from build123d import *

# Parameters (mm, degrees)
SKETCH_1_W                = 44.5
SKETCH_1_H                = 40
EXTRUDE_1_DEPTH           = 9
SKETCH_2_W                = 40.5
SKETCH_2_H                = 7.5
CUT_EXTRUDE_1_DEPTH       = 47.64828507
CUT_EXTRUDE_2_REACH       = 51.611
CUT_EXTRUDE_3_DEPTH       = 50.610986686
HOLE_WIZARD_6_0_6_1_D     = 6
HOLE_WIZARD_6_0_6_1_DEPTH = 9
HOLE_WIZARD_3_0_3_1_D     = 3
HOLE_WIZARD_3_0_3_1_DEPTH = 9
HOLE_WIZARD_2_0_2_1_D     = 2
HOLE_WIZARD_2_0_2_1_DEPTH = 2
HOLE_WIZARD_2_0_2_2_D     = 2
HOLE_WIZARD_2_0_2_2_DEPTH = 44.5
FILLET_1_R                = 1.5
FILLET_2_R                = 2


with BuildPart() as part:
    # 草图1 → 凸台-拉伸1 (new body)
    with BuildSketch(Plane(origin=(0, 9, 0), x_dir=(1, 0, 0), z_dir=(0, 1, 0))):
        Rectangle(SKETCH_1_W, SKETCH_1_H)
    extrude(amount=-EXTRUDE_1_DEPTH)

    # 草图2 → 切除-拉伸1 (cut, through all)
    with BuildSketch(Plane(origin=(0, 0, -20), x_dir=(-1, 0, 0), z_dir=(0, 0, -1))):
        with Locations((0, 5.25)):
            Rectangle(SKETCH_2_W, SKETCH_2_H)
    extrude(amount=-CUT_EXTRUDE_1_DEPTH, mode=Mode.SUBTRACT)

    # 草图3 → 切除-拉伸2 (cut, up to next)
    with BuildSketch(Plane(origin=(22.25, 0, 0), x_dir=(0, 0, -1), z_dir=(1, 0, 0)), mode=Mode.PRIVATE) as cut_extrude_2_sk1:
        with BuildLine():
            Line((14.153311931, 9), (5.846688069, 9))
            ThreePointArc((5.846688069, 9), (10, 7.5), (14.153311931, 9))
        make_face()
    cut_extrude_2_tool1 = extrude(cut_extrude_2_sk1.sketch, amount=-CUT_EXTRUDE_2_REACH, mode=Mode.PRIVATE) & part.part
    add(cut_extrude_2_tool1.solids().sort_by_distance((22.25, 8.39364, -10))[0], mode=Mode.SUBTRACT)

    # 草图4 → 切除-拉伸3 (cut, through all)
    with BuildSketch(Plane.ZY.offset(22.25)):
        with BuildLine():
            Line((-5.846688069, 9), (-14.153311931, 9))
            ThreePointArc((-14.153311931, 9), (-10, 7.5), (-5.846688069, 9))
        make_face()
    extrude(amount=-CUT_EXTRUDE_3_DEPTH, mode=Mode.SUBTRACT)

    # Ø6.0 (6) 直径孔1
    with Locations(Plane(origin=(0, 0, 0), x_dir=(-1, 0, 0), z_dir=(0, -1, 0))):
        with Locations((0, 0), (0, 10), (0, -10)):
            Hole(HOLE_WIZARD_6_0_6_1_D / 2, depth=HOLE_WIZARD_6_0_6_1_DEPTH)

    # Ø3.0 (3) 直径孔1
    with Locations(Plane(origin=(0, 0, 0), x_dir=(-1, 0, 0), z_dir=(0, -1, 0))):
        with Locations((5, 5), (-5, 5), (-5, -5), (5, -5), (5, 15), (-5, 15), (-5, -15), (5, -15), (13.5, 10), (13.5, 0), (13.5, -10), (-13.5, 10), (-13.5, 0), (-13.5, -10)):
            Hole(HOLE_WIZARD_3_0_3_1_D / 2, depth=HOLE_WIZARD_3_0_3_1_DEPTH)

    # Ø2.0 (2) 直径孔1
    with Locations(Plane.ZY.offset(22.25)):
        with Locations((-17.5, 6.5), (2.5, 6.5), (10.4, 7), (17.5, 6.5), (-2.82, 6)):
            Hole(HOLE_WIZARD_2_0_2_1_D / 2, depth=HOLE_WIZARD_2_0_2_1_DEPTH)

    # Ø2.0 (2) 直径孔2
    with Locations(Plane(origin=(22.25, 0, 0), x_dir=(0, 0, -1), z_dir=(1, 0, 0))):
        with Locations((17.5, 6.5), (-2.5, 6.5), (-10.4, 7), (-17.5, 6.5), (2.82, 6)):
            Hole(HOLE_WIZARD_2_0_2_2_D / 2, depth=HOLE_WIZARD_2_0_2_2_DEPTH)

    # 圆角1
    fillet_1_edges = [part.edges().sort_by_distance(p)[0] for p in [
        (22.25, 0, 0),
        (21.25, 9, 20),
        (-21.25, 9, -20),
        (-22.25, 0, 0),
        (21.25, 9, -20),
        (-21.25, 9, 20),
    ]]
    fillet(fillet_1_edges, radius=FILLET_1_R)

    # 圆角2
    fillet_2_edges = [part.edges().sort_by_distance(p)[0] for p in [
        (21.25, 9, -5.846688069),
        (21.25, 9, -14.153311931),
        (-21.25, 9, -5.846688069),
        (-21.25, 9, -14.153311931),
    ]]
    fillet(fillet_2_edges, radius=FILLET_2_R)


solid = part.part
Verification items for the finished model (mm, model axes). A direction names the side the tool comes from. Give positions to 0.01 mm unless a question says otherwise; leave off trailing zeros. Loops run counter-clockwise (first coordinate to the right, second up) from the corner with the lowest first, then second, coordinate; pieces in that order, holes last. Notation, with made-up numbers: (13.25, 33.25) - (72.25, 33.25) arc R34 cw to (72.25, 68.25) - close; hole circle Ø7 at (-9, 65). An arc over 180 degrees is marked (long way). Write item = value, one per line. Start each with the question number.
Q1. Tool access check on faces 1 (the face through (20.25, 5, 0)), 2 (the face through (21, 9, 6)), 3 (the face through (21.2, 8.9, -14.2)). Record the directions out of +Z, -Z, +X, -X, +Y, -Y that give a thin tool (end or side, any length) a straight path to the whole face; none if there is none.
Q2. Cross-section at C-C, the plane z = -9.5. Enter the section's corners in (x, y).
Q3. Cross-section at D-D, the plane x = -5. Enter the section's corners in (y, z).
Q4. Cross-section at A-A, the plane y = 3.75. Enter the section's corners in (x, z).
Q5. Cross-section at B-B, the plane x = 13.5. Enter the section's corners in (y, z).
Q6. Mould release check, pull along Z, two halves, no side actions. Record for faces 4 (the face through (21.26, 8.57, 19.55)), 5 (the face through (-21, 9, -17)), 6 (the face through (12, 1, 0)): released by +Z, released by -Z, zero draft, split by the parting line, or undercut.
Q7. Thickness scan on line 1 (Z direction, x = 5, y = 0.9); line 2 (Z direction, x = -13.5, y = 1.15); line 3 (X direction, y = 7, z = 5.5). Record the ranges inside material, lowest first.
Q8. Depth check by flat-ended pin: P1, Ø20, axis at x = 6.5, z = -1, coming from the +Y side; P2, Ø1.8, axis at x = 5, z = -15, coming from the -Y side. Enter the tip coordinate at first touch or a pass-through.
Answer key:
q1.face_1 = +Z, -Z, +Y
q1.face_2 = +Z, -Z, +X, -X, +Y
q1.face_3 = +X, -X, +Y
q2.outline = (-22.25, 1.5) arc R1.5 ccw to (-20.75, 0) - (-14.91, 0) - (-14.91, 1.5) - (-20.25, 1.5) - (-20.25, 7.52) - (-22.25, 7.52) - close; (-12.09, 0) - (-2.96, 0) - (-2.96, 1.5) - (-12.09, 1.5) - close; (2.96, 0) - (12.09, 0) - (12.09, 1.5) - (2.96, 1.5) - close; (14.91, 0) - (20.75, 0) arc R1.5 ccw to (22.25, 1.5) - (22.25, 7.52) - (20.25, 7.52) - (20.25, 1.5) - (14.91, 1.5) - close
q3.outline = (0, -20) - (1.5, -20) - (1.5, -16.5) - (0, -16.5) - close; (0, -13.5) - (1.5, -13.5) - (1.5, -6.5) - (0, -6.5) - close; (0, -3.5) - (1.5, -3.5) - (1.5, 3.5) - (0, 3.5) - close; (0, 6.5) - (1.5, 6.5) - (1.5, 13.5) - (0, 13.5) - close; (0, 16.5) - (1.5, 16.5) - (1.5, 20) - (0, 20) - close
q4.outline = (-22.25, -20) - (-20.25, -20) - (-20.25, 20) - (-22.25, 20) - close; (20.25, -20) - (22.25, -20) - (22.25, 20) - (20.25, 20) - close
q5.outline = (0, -20) - (1.5, -20) - (1.5, -11.5) - (0, -11.5) - close; (0, -8.5) - (1.5, -8.5) - (1.5, -1.5) - (0, -1.5) - close; (0, 1.5) - (1.5, 1.5) - (1.5, 8.5) - (0, 8.5) - close; (0, 11.5) - (1.5, 11.5) - (1.5, 20) - (0, 20) - close
q6.face_4 = released by +Z
q6.face_5 = zero draft
q6.face_6 = undercut
q7.line_1 = -20 to -16.5, -13.5 to -6.5, -3.5 to 3.5, 6.5 to 13.5, 16.5 to 20
q7.line_2 = -20 to -11.5, -8.5 to -1.5, 1.5 to 8.5, 11.5 to 20
q7.line_3 = -22.25 to -20.25, 20.25 to 22.25
q8.P1 = 1.5
q8.P2 = through
